Design review of the part built by this model. Coordinates are the model's own, in mm. Give positions to 0.01 mm unless a question says otherwise; leave off trailing zeros. Loops run counter-clockwise (first coordinate to the right, second up) from the corner with the lowest first, then second, coordinate; pieces in that order, holes last. Notation, with made-up numbers: (55, -13) -> (59, -13) arc R26 ccw to (59, 10) -> close; hole circle Ø11 at (73, 18). An arc over 180 degrees is marked (long way). Answer as CSV lines item,"result".
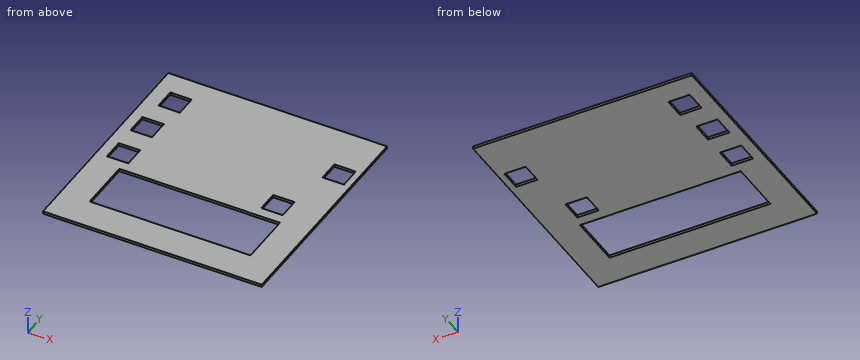
from build123d import *

# Parameters (mm, degrees)
SKETCH_1_W               = 102
SKETCH_1_H               = 106
EXTRUDE_1_DEPTH          = 1.2
CUT_EXTRUDE_2_DEPTH      = 10
CUT_EXTRUDE_2_DEPTH_BACK = 10
SKETCH_2_W               = 75
SKETCH_2_H               = 25
CUT_EXTRUDE_3_DEPTH      = 10
CUT_EXTRUDE_3_DEPTH_BACK = 10
SKETCH_3_W               = 10
SKETCH_3_H               = 10
CUT_EXTRUDE_4_DEPTH      = 10
CUT_EXTRUDE_4_DEPTH_BACK = 10
SKETCH_4_W               = 10
SKETCH_4_H               = 10


with BuildPart() as part:
    # 草图1 → 凸台-拉伸1 (new body)
    with BuildSketch(Plane.XY):
        Rectangle(SKETCH_1_W, SKETCH_1_H)
    extrude(amount=EXTRUDE_1_DEPTH)

    # 草图2 → 切除-拉伸2 (cut, two sides: drawn at the far end of the back side and taken through both)
    with BuildSketch(Plane.XY.offset(1.2).offset(-CUT_EXTRUDE_2_DEPTH_BACK)):
        with Locations((0, -25.5)):
            Rectangle(SKETCH_2_W, SKETCH_2_H)
    extrude(amount=CUT_EXTRUDE_2_DEPTH + CUT_EXTRUDE_2_DEPTH_BACK, mode=Mode.SUBTRACT)

    # 草图3 → 切除-拉伸3 (cut, two sides: drawn at the far end of the back side and taken through both)
    with BuildSketch(Plane.XY.offset(1.2).offset(-CUT_EXTRUDE_3_DEPTH_BACK)):
        with Locations((-41, -3)):
            Rectangle(SKETCH_3_W, SKETCH_3_H)
        with Locations((31, -3)):
            Rectangle(SKETCH_3_W, SKETCH_3_H)
    extrude(amount=CUT_EXTRUDE_3_DEPTH + CUT_EXTRUDE_3_DEPTH_BACK, mode=Mode.SUBTRACT)

    # 草图4 → 切除-拉伸4 (cut, two sides: drawn at the far end of the back side and taken through both)
    with BuildSketch(Plane.XY.offset(1.2).offset(-CUT_EXTRUDE_4_DEPTH_BACK)):
        with Locations((-41, 17)):
            Rectangle(SKETCH_4_W, SKETCH_4_H)
        with Locations((-39, 37)):
            Rectangle(SKETCH_4_W, SKETCH_4_H)
        with Locations((43, 27)):
            Rectangle(SKETCH_4_W, SKETCH_4_H)
    extrude(amount=CUT_EXTRUDE_4_DEPTH + CUT_EXTRUDE_4_DEPTH_BACK, mode=Mode.SUBTRACT)


solid = part.part
Q1. To check wall thickness, follow probe 1 along Y at (x, z) = (35, 0.25); probe 2 along X at (y, z) = (-2, 1.05); probe 3 along X at (y, z) = (21, 0.7). State the ranges of each line that lie inside material, in increasing order. Write a range as from..to.
Filled sheet:
probe 1,"y = -53..-38, -13..-8, 2..53"
probe 2,"x = -51..-46, -36..26, 36..51"
probe 3,"x = -51..-46, -36..51"
Q2. We need section B-B, the plane z = 0.45. State the section outline as (x, y) points, and give its area (3 significant figures).
Filled sheet:
outline,"(-51, -53) -> (51, -53) -> (51, 53) -> (-51, 53) -> close; hole (-46, -8) -> (-36, -8) -> (-36, 2) -> (-46, 2) -> close; hole (-46, 12) -> (-36, 12) -> (-36, 22) -> (-46, 22) -> close; hole (-44, 32) -> (-34, 32) -> (-34, 42) -> (-44, 42) -> close; hole (-37.5, -38) -> (37.5, -38) -> (37.5, -13) -> (-37.5, -13) -> close; hole (26, -8) -> (36, -8) -> (36, 2) -> (26, 2) -> close; hole (38, 22) -> (48, 22) -> (48, 32) -> (38, 32) -> close"
area,"8,440 mm^2"
Q3. We need section D-D, the plane x = -17. State the section outline as (y, z) points.
Filled sheet:
outline,"(-53, 0) -> (-38, 0) -> (-38, 1.2) -> (-53, 1.2) -> close; (-13, 0) -> (53, 0) -> (53, 1.2) -> (-13, 1.2) -> close"
Q4. We need section A-A, the plane y = -19. State the section outline as (x, z) points, and give its area (3 significant figures).
Filled sheet:
outline,"(-51, 0) -> (-37.5, 0) -> (-37.5, 1.2) -> (-51, 1.2) -> close; (37.5, 0) -> (51, 0) -> (51, 1.2) -> (37.5, 1.2) -> close"
area,"32.4 mm^2"
Q5. We need section C-C, the plane y = -6.5. State the section outline as (x, z) points.
Filled sheet:
outline,"(-51, 0) -> (-46, 0) -> (-46, 1.2) -> (-51, 1.2) -> close; (-36, 0) -> (26, 0) -> (26, 1.2) -> (-36, 1.2) -> close; (36, 0) -> (51, 0) -> (51, 1.2) -> (36, 1.2) -> close"
